from build123d import *

# Parameters (mm, degrees)
SKETCH1_R           = 4
BOSS_EXTRUDE1_DEPTH = 40
CUT_EXTRUDE1_START  = 2.5
CUT_EXTRUDE1_DEPTH  = 38.898019753
CHAMFER1_SIZE       = 0.5
SKETCH3_W           = 0.6
SKETCH3_H           = 1
BOSS_EXTRUDE2_DEPTH = 10
CIRPATTERN1_COUNT   = 10


with BuildPart() as part:
    # Sketch1 → Boss-Extrude1 (new body)
    with BuildSketch(Plane.XY):
        Circle(SKETCH1_R)
    extrude(amount=BOSS_EXTRUDE1_DEPTH)

    # Sketch2 → Cut-Extrude1 (cut, through all)
    with BuildSketch(Plane(origin=(0, 0, 0), x_dir=(1, 0, 0), z_dir=(0, 1, 0)).offset(CUT_EXTRUDE1_START)):
        with BuildLine():
            Line((1.5, 0), (1.5, -4))
            ThreePointArc((1.5, -4), (0, -5.5), (-1.5, -4))
            Line((-1.5, -4), (-1.5, 0))
            ThreePointArc((-1.5, 0), (0, 1.5), (1.5, 0))
        make_face()
    extrude(amount=CUT_EXTRUDE1_DEPTH, mode=Mode.SUBTRACT)

    # Chamfer1
    chamfer1_edges = [part.edges().sort_by_distance(p)[0] for p in [
        (-2.236067977, -3.31662479, 0),
    ]]
    chamfer(chamfer1_edges, length=CHAMFER1_SIZE)

    # Sketch3 → Boss-Extrude2 (add)
    with BuildSketch(Plane.XY.offset(40)):
        with Locations((0, 4)):
            Rectangle(SKETCH3_W, SKETCH3_H)
    boss_extrude2 = extrude(amount=-BOSS_EXTRUDE2_DEPTH)

    # CirPattern1: Boss-Extrude2 ×10 about axis
    cirpattern1_axis = Axis((0, 0, 0), (0, 0, 1))
    for i in range(1, CIRPATTERN1_COUNT):
        add(boss_extrude2.rotate(cirpattern1_axis, i * 360 / CIRPATTERN1_COUNT))


solid = part.part
Read the model definition and answer for the solid it produces. Units are mm, in the model's axes. A direction names the side the tool comes from. Round coordinates to 2 decimals unless told otherwise and drop trailing zeros. Order: outer loops, then holes, each group sorted by start corner. A loop starts at its lowest first (then second) coordinate and runs counter-clockwise, first axis right, second up.
1) The mould has two halves that part along X. Classify faces 1 (the face through (0, 3.2, 5.5)), 2 (the face through (-0.14, -3.633, 0.135)), 3 (the face through (0, 0, 0)): released by +X, released by -X, zero draft, split by the parting line, or undercut.
2) Straight lines are drawn through the part: L1, parallel to X at y = -3.5, z = 34.5; L2, parallel to Y at x = -1.5, z = 7.5; L3, parallel to Y at x = -0.25, z = 21. For each, find the intervals that lie inside material, in ascending order.
3) Flat-ended cylindrical pins translate along their axes: pin 1 (0.6 mm diameter, centred on y = 3, z = 2.5, fed in from +X); pin 2 (0.5 mm diameter, centred on x = 4, y = -1, fed in from -Z); pin 3 (5 mm diameter, centred on y = -1.5, z = 32.5, fed in from -X). Find the tip coordinate at first contact, or state that the pin passes through.
4) The part is cut by section A-A on z = 23. Write down the section's boundary in (x, y), plus the area to 3 significant figures.
5) For faces 4 (the face through (-3.2, -2.4, 20)), 5 (the face through (0, 2.5, 3)), 6 (the face through (0, 0, 40)), determine the directions among +Z, -Z, +X, -X, +Y, -Y from which every point of the face is accessible in a straight line to the end or side of a thin tool.
Resolved:
1. face 1: undercut
1. face 2: split by the parting line
1. face 3: zero draft
2. L1: x = -2.84 to -2.17, -1.94 to 1.94, 2.17 to 2.84
2. L2: y = -3.71 to 3.71
2. L3: y = -3.99 to 3.99
3. pin 1: stops at x = 2.95
3. pin 2: stops at z = 0.37
3. pin 3: stops at x = -4.37
4. outline: circle Ø8 at (0, 0)
4. area: 50.3 mm2
5. face 4: -Z
5. face 5: -Z, +Y
5. face 6: +Z, +X, -X, +Y, -Y
